```python
from build123d import *

# Parameters (mm, degrees)
BOSS_EXTRUDE1_DEPTH = 50.2
CUT_EXTRUDE2_DEPTH  = 44.2
SKETCH3_W           = 20.2
SKETCH3_H           = 10.1
BOSS_EXTRUDE2_DEPTH = 5
SKETCH4_R           = 1.05
CUT_EXTRUDE3_DEPTH  = 11
SKETCH5_R           = 4
SKETCH5_R_2         = 7.5
CUT_EXTRUDE4_DEPTH  = 11
SKETCH6_R           = 4
BOSS_EXTRUDE3_DEPTH = 5
SKETCH7_R           = 4
SKETCH7_R_2         = 1.05
CUT_EXTRUDE5_DEPTH  = 16
SKETCH8_R           = 7.5
CUT_EXTRUDE6_DEPTH  = 11
SKETCH9_R           = 4
BOSS_EXTRUDE4_DEPTH = 5
SKETCH11_W          = 20.2
SKETCH11_H          = 50.2
BOSS_EXTRUDE5_DEPTH = 3
SKETCH12_R          = 3
SKETCH12_R_2        = 1.55
CUT_EXTRUDE8_DEPTH  = 23
SKETCH13_W          = 20.7
SKETCH13_H          = 20.2
BOSS_EXTRUDE6_DEPTH = 6
SKETCH14_R          = 1.55
CUT_EXTRUDE9_DEPTH  = 6
SKETCH15_R          = 1.55
CUT_EXTRUDE10_DEPTH = 6
FILLET1_R           = 10
FILLET2_R           = 10
FILLET3_R           = 10


with BuildPart() as part:
    # Sketch1 → Boss-Extrude1 (new body)
    with BuildSketch(Plane.XY):
        with BuildLine():
            Line((-10.1, 0), (-10.1, -20))
            Line((-10.1, -20), (10.1, -20))
            Line((10.1, -20), (10.1, 0))
            ThreePointArc((10.1, 0), (0, 10.1), (-10.1, 0))
        make_face()
    extrude(amount=BOSS_EXTRUDE1_DEPTH)

    # Sketch2 → Cut-Extrude2 (cut)
    with BuildSketch(Plane.ZY.offset(10.1)):
        Polygon((5, -10), (5, -17), (45.2, -17), (45.2, -10), (45.2, 11.866817026), (5, 11.866817026), align=None)
    extrude(amount=-CUT_EXTRUDE2_DEPTH, mode=Mode.SUBTRACT)

    # Sketch3 → Boss-Extrude2 (add)
    with BuildSketch(Plane.XY.offset(50.2)):
        with Locations((0, 5.05)):
            Rectangle(SKETCH3_W, SKETCH3_H)
    extrude(amount=-BOSS_EXTRUDE2_DEPTH)

    # Sketch4 → Cut-Extrude3 (cut, symmetric)
    with BuildSketch(Plane.XY.offset(50.2)):
        with Locations((-7.85, 7.85)):
            Circle(SKETCH4_R)
        with Locations((7.85, 7.85)):
            Circle(SKETCH4_R)
        with Locations((-7.85, -7.85)):
            Circle(SKETCH4_R)
        with Locations((7.85, -7.85)):
            Circle(SKETCH4_R)
        with Locations((0, 7.85)):
            Circle(SKETCH4_R)
        with Locations((0, -7.85)):
            Circle(SKETCH4_R)
        with Locations((-7.85, 0)):
            Circle(SKETCH4_R)
        with Locations((7.85, 0)):
            Circle(SKETCH4_R)
    extrude(amount=CUT_EXTRUDE3_DEPTH, both=True, mode=Mode.SUBTRACT)

    # Sketch5 → Cut-Extrude4 (cut, symmetric)
    with BuildSketch(Plane.XY.offset(50.2)):
        Circle(SKETCH5_R)
        with Locations((0, 12.82)):
            Circle(SKETCH5_R_2)
    extrude(amount=CUT_EXTRUDE4_DEPTH, both=True, mode=Mode.SUBTRACT)

    # Sketch6 → Boss-Extrude3 (add)
    with BuildSketch(Plane.XY.offset(50.2)):
        Circle(SKETCH6_R)
    extrude(amount=-BOSS_EXTRUDE3_DEPTH)

    # Sketch7 → Cut-Extrude5 (cut, symmetric)
    with BuildSketch(Plane(origin=(0, 0, 0), x_dir=(-1, 0, 0), z_dir=(0, 0, -1))):
        with Locations(Location((0, 0, 0), (0, 0, 90))):
            Circle(SKETCH7_R)
        with Locations(Location((0, 7, 0), (0, 0, 90))):
            Circle(SKETCH7_R_2)
        with Locations(Location((-4.949747468, 4.949747468, 0), (0, 0, 90))):
            Circle(SKETCH7_R_2)
        with Locations(Location((-7, 0, 0), (0, 0, 90))):
            Circle(SKETCH7_R_2)
        with Locations(Location((-4.949747468, -4.949747468, 0), (0, 0, 90))):
            Circle(SKETCH7_R_2)
        with Locations(Location((0, -7, 0), (0, 0, 90))):
            Circle(SKETCH7_R_2)
        with Locations(Location((4.949747468, -4.949747468, 0), (0, 0, 90))):
            Circle(SKETCH7_R_2)
        with Locations(Location((7, 0, 0), (0, 0, 90))):
            Circle(SKETCH7_R_2)
        with Locations(Location((4.949747468, 4.949747468, 0), (0, 0, 90))):
            Circle(SKETCH7_R_2)
    extrude(amount=CUT_EXTRUDE5_DEPTH, both=True, mode=Mode.SUBTRACT)

    # Sketch8 → Cut-Extrude6 (cut, symmetric)
    with BuildSketch(Plane(origin=(0, 0, 0), x_dir=(-1, 0, 0), z_dir=(0, 0, -1))):
        with Locations((0, 12.82)):
            Circle(SKETCH8_R)
    extrude(amount=CUT_EXTRUDE6_DEPTH, both=True, mode=Mode.SUBTRACT)

    # Sketch9 → Boss-Extrude4 (add)
    with BuildSketch(Plane(origin=(0, 0, 0), x_dir=(-1, 0, 0), z_dir=(0, 0, -1))):
        Circle(SKETCH9_R)
    extrude(amount=-BOSS_EXTRUDE4_DEPTH)

    # Sketch11 → Boss-Extrude5 (add)
    with BuildSketch(Plane(origin=(0, -20, 0), x_dir=(-1, 0, 0), z_dir=(0, -1, 0))):
        with Locations((0, -25.1)):
            Rectangle(SKETCH11_W, SKETCH11_H)
    extrude(amount=BOSS_EXTRUDE5_DEPTH)

    # Sketch12 → Cut-Extrude8 (cut)
    with BuildSketch(Plane(origin=(0, -17, 0), x_dir=(1, 0, 0), z_dir=(0, 1, 0))):
        with Locations(Location((0, -25.1, 0), (0, 0, 270))):
            Circle(SKETCH12_R)
        with Locations(Location((-5.084097757, -20.015902243, 0), (0, 0, 270))):
            Circle(SKETCH12_R_2)
        with Locations(Location((5.084097757, -20.015902243, 0), (0, 0, 270))):
            Circle(SKETCH12_R_2)
        with Locations(Location((5.084097757, -30.184097757, 0), (0, 0, 270))):
            Circle(SKETCH12_R_2)
        with Locations(Location((-5.084097757, -30.184097757, 0), (0, 0, 270))):
            Circle(SKETCH12_R_2)
    extrude(amount=-CUT_EXTRUDE8_DEPTH, mode=Mode.SUBTRACT)

    # Sketch13 → Boss-Extrude6 (add)
    with BuildSketch(Plane(origin=(0, -23, 0), x_dir=(-1, 0, 0), z_dir=(0, -1, 0))):
        with Locations((20.45, -25.1)):
            Rectangle(SKETCH13_W, SKETCH13_H)
        with Locations((-20.45, -25.1)):
            Rectangle(SKETCH13_W, SKETCH13_H)
    extrude(amount=-BOSS_EXTRUDE6_DEPTH)

    # Sketch14 → Cut-Extrude9 (cut)
    with BuildSketch(Plane.XZ.offset(23)):
        with Locations(Location((-15.254097757, 20.015902243, 0), (0, 0, 270))):
            Circle(SKETCH14_R)
        with Locations(Location((-15.254097757, 30.184097757, 0), (0, 0, 90))):
            Circle(SKETCH14_R)
        with Locations(Location((15.254097757, 30.184097757, 0), (0, 0, 270))):
            Circle(SKETCH14_R)
        with Locations(Location((15.254097757, 20.015902243, 0), (0, 0, 90))):
            Circle(SKETCH14_R)
    extrude(amount=-CUT_EXTRUDE9_DEPTH, mode=Mode.SUBTRACT)

    # Sketch15 → Cut-Extrude10 (cut)
    with BuildSketch(Plane(origin=(0, -23, 0), x_dir=(-1, 0, 0), z_dir=(0, -1, 0))):
        with Locations(Location((-5.084097757, -9.845902243, 0), (0, 0, 90))):
            Circle(SKETCH15_R)
        with Locations(Location((5.084097757, -9.845902243, 0), (0, 0, 270))):
            Circle(SKETCH15_R)
        with Locations(Location((-5.084097757, -40.354097757, 0), (0, 0, 270))):
            Circle(SKETCH15_R)
        with Locations(Location((5.084097757, -40.354097757, 0), (0, 0, 90))):
            Circle(SKETCH15_R)
    extrude(amount=-CUT_EXTRUDE10_DEPTH, mode=Mode.SUBTRACT)

    # Fillet1
    fillet1_edges = [part.edges().sort_by_distance(p)[0] for p in [
        (-10.1, -20, 35.2),
    ]]
    fillet(fillet1_edges, radius=FILLET1_R)

    # Fillet2
    fillet2_edges = [part.edges().sort_by_distance(p)[0] for p in [
        (-10.1, -20, 15),
    ]]
    fillet(fillet2_edges, radius=FILLET2_R)

    # Fillet3
    fillet3_edges = [part.edges().sort_by_distance(p)[0] for p in [
        (10.1, -20, 35.2),
        (10.1, -20, 15),
    ]]
    fillet(fillet3_edges, radius=FILLET3_R)


solid = part.part
```
Check sheet for the modelled part. Datum: model origin and axes. Units: mm. A direction names the side the tool comes from. Coordinates: 2 decimals unless noted, no trailing zeros. Write each loop counter-clockwise with the first axis right and the second up, starting at its lowest first coordinate (ties: lowest second). Pieces come first, ordered by that corner, then holes. Notation, with made-up numbers: (78.25, 70) -> (104.25, 70) arc R15 cw to (104.25, 94) -> close; hole circle Ø5 at (78, 41). An arc over 180 degrees is marked (long way). Use a Markdown table: item, result.
1. Sectioned sample at A-A (y = -14). Enter the section's corners in (x, z), plus the area to 3 significant figures.
Reported:
| item | result |
|---|---|
| outline | (-10.1, 0) -> (10.1, 0) -> (10.1, 5) -> (-10.1, 5) -> close; (-10.1, 45.2) -> (10.1, 45.2) -> (10.1, 50.2) -> (-10.1, 50.2) -> close |
| area | 202 mm2 |
2. Sectioned sample at B-B (z = 9). Enter the section's corners in (x, y), plus the area to 3 significant figures.
Reported:
| item | result |
|---|---|
| outline | (-10.93, -23) -> (-6.38, -23) -> (-6.38, -17) -> (-10.93, -17) -> close; (-3.79, -23) -> (3.79, -23) -> (3.79, -17) -> (-3.79, -17) -> close; (6.38, -23) -> (10.93, -23) -> (10.93, -17) -> (6.38, -17) -> close |
| area | 100 mm2 |
3. Tool access check on faces 1 (the cylindrical face through (7.89, 0.56, 2.46)), 2 (the flat face through (26, -20, 35.2)), 3 (the flat face through (-10.1, -11, 3)). Record the directions out of +Z, -Z, +X, -X, +Y, -Y that give a thin tool (end or side, any length) a straight path to the whole face; none if there is none.
Reported:
| item | result |
|---|---|
| face 1 | -Z |
| face 2 | +Z, +X, +Y, -Y |
| face 3 | -Z, -X, +Y, -Y |
4. Sectioned sample at D-D (y = -19). Give the number of separate pieces and of enclosed holes in the cut face, plus the area to 3 significant figures.
Reported:
| item | result |
|---|---|
| separate pieces | 1 |
| enclosed holes | 13 |
| area | 1,820 mm2 |
5. Go/stop test with flat-tipped pins: pin 1 Ø4 at (x, z) = (-5.08, 9.85) entering from +Y; pin 2 Ø6.5 at (x, y) = (-25, -19.5) entering from -Z; pin 3 Ø2.5 at (x, y) = (7.85, -7.85) entering from +Z; pin 4 Ø1.9 at (x, y) = (-7, 0) entering from -Z. Record where each tip stops, or that it passes through.
Reported:
| item | result |
|---|---|
| pin 1 | stops at y = -17 |
| pin 2 | stops at z = 15 |
| pin 3 | stops at z = 50.2 |
| pin 4 | stops at z = 45.2 |
6. Sectioned sample at C-C (z = 27). Enter the section's corners in (x, y), plus the area to 3 significant figures.
Reported:
| item | result |
|---|---|
| outline | (-30.8, -23) -> (-2.32, -23) -> (-2.32, -17) -> (-30.8, -17) -> close; (2.32, -23) -> (30.8, -23) -> (30.8, -17) -> (2.32, -17) -> close |
| area | 342 mm2 |
7. Release check for a two-part mould opening along X. For faces 4 (the flat face through (10.1, -6, 48)), 5 (the cylindrical face through (-16.63, -20.04, 19.3)), 6 (the flat face through (-10.1, -6, 48)), 7 (the flat face through (9, 10.1, 48)) record: pulls with the +X half, pulls with the -X half, needs draft (parallel to the pull), parting line crosses it, or undercut.
Reported:
| item | result |
|---|---|
| face 4 | pulls with the +X half |
| face 5 | undercut |
| face 6 | pulls with the -X half |
| face 7 | needs draft |
8. Scan lines: line 1 along Z through (x, y) = (-6, 6.5); line 2 along Y through (x, z) = (-7, 46); line 3 along Y through (x, z) = (22, 35). Record each from-to range of solid material in increasing order.
Reported:
| item | result |
|---|---|
| line 1 | z = 0 to 5, 45.2 to 50.2 |
| line 2 | y = -23 to -8.47, -7.23 to -0.62, 0.62 to 7.23, 8.47 to 10.1 |
| line 3 | y = -23 to -17 |
